Read the model definition and answer for the solid it produces. Units are mm, in the model's axes. Coordinates: 2 decimals unless noted, no trailing zeros. Loops run counter-clockwise (first coordinate to the right, second up) from the corner with the lowest first, then second, coordinate; pieces in that order, holes last.
from build123d import *

# Parameters (mm, degrees)
SKETCH_1_W      = 99.9
SKETCH_1_H      = 23.7
SKETCH_1_R      = 1
SKETCH_1_W_2    = 29.5
SKETCH_1_H_2    = 10
EXTRUDE_1_DEPTH = 1.6


with BuildPart() as part:
    # 草图1 → 凸台-拉伸1 (new body)
    with BuildSketch(Plane.XY):
        with Locations((49.95, -11.85)):
            Rectangle(SKETCH_1_W, SKETCH_1_H)
        with Locations((39.5, -2.9)):
            Circle(SKETCH_1_R, mode=Mode.SUBTRACT)
        with Locations((35.4, -8.1)):
            Circle(SKETCH_1_R, mode=Mode.SUBTRACT)
        with Locations((39.5, -13.2)):
            Circle(SKETCH_1_R, mode=Mode.SUBTRACT)
        with Locations(Location((60.4, -2.9, 0), (0, 0, 180))):
            Circle(SKETCH_1_R, mode=Mode.SUBTRACT)
        with Locations(Location((64.5, -8.1, 0), (0, 0, 180))):
            Circle(SKETCH_1_R, mode=Mode.SUBTRACT)
        with Locations(Location((60.4, -13.2, 0), (0, 0, 180))):
            Circle(SKETCH_1_R, mode=Mode.SUBTRACT)
        with Locations((18.65, -10.1)):
            Rectangle(SKETCH_1_W_2, SKETCH_1_H_2, mode=Mode.SUBTRACT)
        with Locations((81.25, -10.1)):
            Rectangle(SKETCH_1_W_2, SKETCH_1_H_2, mode=Mode.SUBTRACT)
    extrude(amount=EXTRUDE_1_DEPTH)


solid = part.part
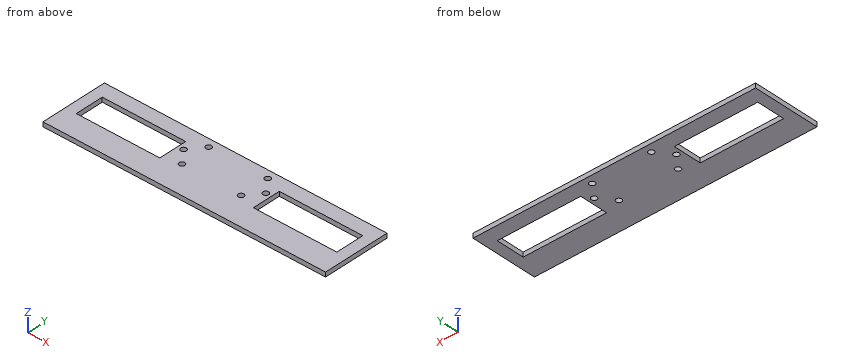
Item 1: Given pin 1 (2.5 mm diameter, centred on x = 35.4, y = -8.1, fed in from -Z), flat-ended and moving along its own axis, determine where the tip first touches the part or whether it passes through.
Numbers:
pin 1: stops at z = 0
Item 2: A cutting plane is placed at C-C on x = 92. Determine the outline of the cut face in (y, z), then the cut area to 3 significant figures.
Numbers:
outline: (-23.7, 0) - (-15.1, 0) - (-15.1, 1.6) - (-23.7, 1.6) - close; (-5.1, 0) - (0, 0) - (0, 1.6) - (-5.1, 1.6) - close
area: 21.9 mm2
Item 3: A cutting plane is placed at B-B on x = 60.4. Determine the outline of the cut face in (y, z).
Numbers:
outline: (-23.7, 0) - (-14.2, 0) - (-14.2, 1.6) - (-23.7, 1.6) - close; (-12.2, 0) - (-3.9, 0) - (-3.9, 1.6) - (-12.2, 1.6) - close; (-1.9, 0) - (0, 0) - (0, 1.6) - (-1.9, 1.6) - close
Item 4: A cutting plane is placed at A-A on z = 1.1. Give the number of separate pieces and of enclosed holes in the cut face, then the cut area to 3 significant figures.
Numbers:
separate pieces: 1
enclosed holes: 8
area: 1,760 mm2
Item 5: Find the intervals of material crossed by line 1 along X through (y, z) = (-8, 0.7); line 2 along Y through (x, z) = (39.5, 1.05); line 3 along Y through (x, z) = (9, 0.3), in increasing order.
Numbers:
line 1: x = 0 to 3.9, 33.4 to 34.41, 36.39 to 63.51, 65.49 to 66.5, 96 to 99.9
line 2: y = -23.7 to -14.2, -12.2 to -3.9, -1.9 to 0
line 3: y = -23.7 to -15.1, -5.1 to 0
Item 6: A cutting plane is placed at D-D on y = -8.1. Determine the outline of the cut face in (x, z).
Numbers:
outline: (0, 0) - (3.9, 0) - (3.9, 1.6) - (0, 1.6) - close; (33.4, 0) - (34.4, 0) - (34.4, 1.6) - (33.4, 1.6) - close; (36.4, 0) - (63.5, 0) - (63.5, 1.6) - (36.4, 1.6) - close; (65.5, 0) - (66.5, 0) - (66.5, 1.6) - (65.5, 1.6) - close; (96, 0) - (99.9, 0) - (99.9, 1.6) - (96, 1.6) - close
